from build123d import *

# Parameters (mm, degrees)
BOSS_EXTRUDE1_DEPTH                  = 50
TAP_DRILL_FOR_M5X0_8_TAP1_AT_2_COUNT = 2
TAP_DRILL_FOR_M5X0_8_TAP1_AT_2_PITCH = 19.5
TAP_DRILL_FOR_M5X0_8_TAP1_AT_3_COUNT = 2
TAP_DRILL_FOR_M5X0_8_TAP1_AT_3_PITCH = 39
CUT_EXTRUDE1_DEPTH                   = 20


with BuildPart() as part:
    # Sketch1 → Boss-Extrude1 (new body, symmetric)
    with BuildSketch(Plane(origin=(0, 0, 0), x_dir=(0, 0, -1), z_dir=(1, 0, 0))):
        Polygon((9, 19), (46, 19), (43, 25), (55, 25), (55, 0), (0, 0), (0, 25), (12, 25), align=None)
    extrude(amount=BOSS_EXTRUDE1_DEPTH, both=True)

    # Sketch5 → Tap Drill for M5x0.8 Tap1 (revolve, cut)
    with BuildSketch(Plane(origin=(50, 8, -8), x_dir=(0, 0, -1), z_dir=(0, 1, 0))):
        Polygon((0, 0), (0, 8.401721238), (2, 7.2), (2, 0), align=None)
    tap_drill_for_m5x0_8_tap1 = revolve(axis=Axis((56.35, 8, -8), (-1, 0, 0)), mode=Mode.SUBTRACT)

    # Tap Drill for M5x0.8 Tap1 at 2: Tap Drill for M5x0.8 Tap1 ×2
    with Locations(*[(0, 0, -i * TAP_DRILL_FOR_M5X0_8_TAP1_AT_2_PITCH) for i in range(1, TAP_DRILL_FOR_M5X0_8_TAP1_AT_2_COUNT)]):
        add(tap_drill_for_m5x0_8_tap1, mode=Mode.SUBTRACT)

    # Tap Drill for M5x0.8 Tap1 at 3: Tap Drill for M5x0.8 Tap1 ×2
    with Locations(*[(0, 0, -i * TAP_DRILL_FOR_M5X0_8_TAP1_AT_3_PITCH) for i in range(1, TAP_DRILL_FOR_M5X0_8_TAP1_AT_3_COUNT)]):
        add(tap_drill_for_m5x0_8_tap1, mode=Mode.SUBTRACT)

    # Mirror2: Tap Drill for M5x0.8 Tap1 across plane
    add(tap_drill_for_m5x0_8_tap1.mirror(Plane(origin=(0, 0, 0), x_dir=(0, 0, 1), z_dir=(1, 0, 0))), mode=Mode.SUBTRACT)

    # Mirror2 copy 1 sketch → Mirror2 copy 1 (revolve, cut)
    with BuildSketch(Plane(origin=(-50, 8, -27.5), x_dir=(0, 0, -1), z_dir=(0, 1, 0))):
        Polygon((0, 0), (0, -8.401721238), (2, -7.2), (2, 0), align=None)
    revolve(axis=Axis((-56.35, 8, -27.5), (-1, 0, 0)), mode=Mode.SUBTRACT)

    # Mirror2 copy 2 sketch → Mirror2 copy 2 (revolve, cut)
    with BuildSketch(Plane(origin=(-50, 8, -47), x_dir=(0, 0, -1), z_dir=(0, 1, 0))):
        Polygon((0, 0), (0, -8.401721238), (2, -7.2), (2, 0), align=None)
    revolve(axis=Axis((-56.35, 8, -47), (-1, 0, 0)), mode=Mode.SUBTRACT)

    # Sketch6 → Cut-Extrude1 (cut, through all)
    with BuildSketch(Plane(origin=(0, 19, 0), x_dir=(1, 0, 0), z_dir=(0, 1, 0))):
        with BuildLine():
            Line((-35, 39), (35, 39))
            ThreePointArc((35, 39), (38.535533906, 37.535533906), (40, 34))
            Line((40, 34), (40, 21))
            ThreePointArc((40, 21), (38.535533906, 17.464466094), (35, 16))
            Line((35, 16), (-35, 16))
            ThreePointArc((-35, 16), (-38.535533906, 17.464466094), (-40, 21))
            Line((-40, 21), (-40, 34))
            ThreePointArc((-40, 34), (-38.535533906, 37.535533906), (-35, 39))
        make_face()
    extrude(amount=-CUT_EXTRUDE1_DEPTH, mode=Mode.SUBTRACT)


solid = part.part
Input: part model. Units: mm. Frame: model coordinates. A direction names the side the tool comes from. Round coordinates to 2 decimals unless told otherwise and drop trailing zeros. Write each loop counter-clockwise with the first axis right and the second up, starting at its lowest first coordinate (ties: lowest second). Pieces come first, ordered by that corner, then holes.
1) Ray query, L1, parallel to Z at x = 47.25, y = 8; L2, parallel to Y at x = -45, z = -47; L3, parallel to Z at x = -30, y = 9.75. Return the intervals inside material, ascending.
2) Reachability of faces 4 (the cylindrical face through (38, 10, -38)), 5 (the flat face through (1, 19, -15)), 6 (the cylindrical face through (-46.45, 6.648, -45.526)) from +Z, -Z, +X, -X, +Y, -Y: full face, straight path, thin tool, end or side. Return the list, or none.
3) Draft query along Y for faces 1 (the cylindrical face through (-46, 8, -6)), 2 (the flat face through (1, 13, -55)), 3 (the flat face through (1, 0, -40)). Return one class per face: pulls with the +Y half, pulls with the -Y half, needs draft (parallel to the pull), parting line crosses it, or undercut.
4) Cut plane C-C (y = 4). Return the cut outline in (x, z), then the cut area to 3 significant figures.
5) Contact query for flat-ended pins moving along their axis: P1, Ø3, axis at y = 8, z = -47, coming from the +X side; P2, Ø2.5, axis at y = 8, z = -27.5, coming from the -X side. Output: stop coordinate, or through.
6) Cut plane B-B (x = -31). Return the cut outline in (y, z).
7) Cut plane A-A (z = -37). Return the cut outline in (x, y), then the cut area to 3 significant figures.
Geometry says:
1. L1: z = -55 to -49, -45 to -29.5, -25.5 to -10, -6 to 0
1. L2: y = 0 to 6, 10 to 25
1. L3: z = -55 to -39, -16 to 0
2. face 4: +Y, -Y
2. face 5: +X, -X
2. face 6: -X
3. face 1: undercut
3. face 2: needs draft
3. face 3: pulls with the -Y half
4. outline: (-50, -55) - (50, -55) - (50, 0) - (-50, 0) - close; hole (-40, -34) arc R5 ccw to (-35, -39) - (35, -39) arc R5 ccw to (40, -34) - (40, -21) arc R5 ccw to (35, -16) - (-35, -16) arc R5 ccw to (-40, -21) - close
4. area: 3,680 mm2
5. P1: stops at x = 42.5
5. P2: stops at x = -42.35
6. outline: (0, -55) - (25, -55) - (25, -43) - (19, -46) - (19, -39) - (0, -39) - close; (0, -16) - (19, -16) - (19, -9) - (25, -12) - (25, 0) - (0, 0) - close
7. outline: (-50, 0) - (-39, 0) - (-39, 19) - (-50, 19) - close; (39, 0) - (50, 0) - (50, 19) - (39, 19) - close
7. area: 418 mm2
